The figure shows three views and two pictorial views of one solid part (mm, origin at its lowest corner). Answer the questions. Coordinates: 2 decimals unless noted, no trailing zeros. Write each loop counter-clockwise with the first axis right and the second up, starting at its lowest first coordinate (ties: lowest second). Pieces come first, ordered by that corner, then holes. Notation, with made-up numbers: (24, 57) - (41, 57) arc R11 cw to (41, 71) - close; hole circle Ø3 at (-32.5, -38). An arc over 180 degrees is marked (long way). Use a Markdown table: item, result. Add a question column.
(1) Given pin 1 Ø0.5 at (x, y) = (20.5, 0.5) entering from -Z; pin 2 Ø2.5 at (x, z) = (32.4, 18.17) entering from +Y; pin 3 Ø1.3 at (x, z) = (1.84, 1.84) entering from -Y; pin 4 Ø2 at (y, z) = (1.5, 2) entering from -X, each flat-ended and moving along its own axis, determine where each tip first touches the part or whether it passes through.
(2) The part is cut by section B-B, the plane x = 13. Give the vertices of the cut face in (y, z).
(3) The part is cut by section A-A, the plane y = 0.6. Give the vertices of the cut face in (x, z), then the cut area to 3 significant figures.
(4) Find the intervals of material crossed by line 1 (X direction, y = 0.4, z = 1) (1 decimal); line 2 (X direction, y = 0.6, z = 2.25) (1 decimal); line 3 (Y direction, x = 7, z = 12), in increasing order. Write a range as from..to.
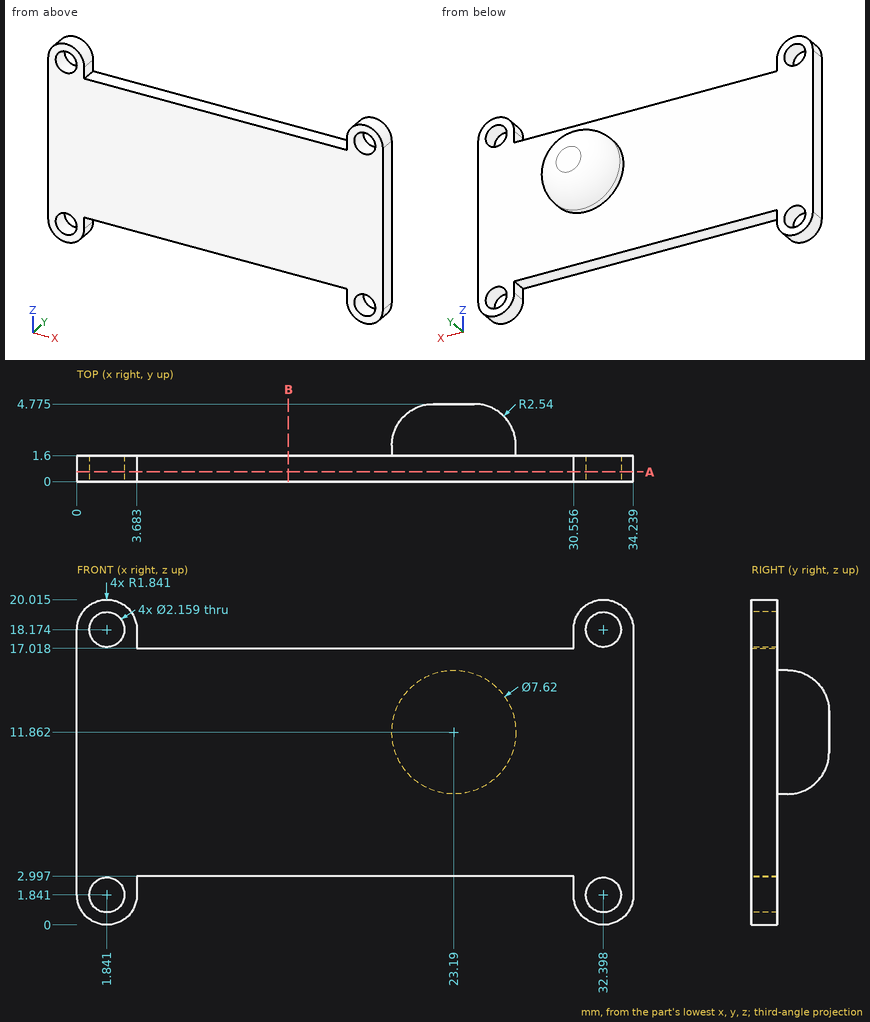
Model answer:
| question | item | result |
|---|---|---|
| 1 | pin 1 | z = 3 |
| 1 | pin 2 | y = 1.6 |
| 1 | pin 3 | through |
| 1 | pin 4 | x = 0 |
| 2 | outline | (0, 3) - (1.6, 3) - (1.6, 17.02) - (0, 17.02) - close |
| 3 | outline | (0, 1.84) arc R1.84 ccw to (3.68, 1.84) - (3.68, 3) - (30.56, 3) - (30.56, 1.84) arc R1.84 ccw to (34.24, 1.84) - (34.24, 18.17) arc R1.84 ccw to (30.56, 18.17) - (30.56, 17.02) - (3.68, 17.02) - (3.68, 18.17) arc R1.84 ccw to (0, 18.17) - close; hole circle Ø2.16 at (1.84, 1.84); hole circle Ø2.16 at (1.84, 18.17); hole circle Ø2.16 at (32.4, 1.84); hole circle Ø2.16 at (32.4, 18.17) |
| 3 | area | 504 mm^2 |
| 4 | line 1 | 0.2..1.2, 2.5..3.5, 30.8..31.7, 33.1..34 |
| 4 | line 2 | 0..0.8, 2.8..3.7, 30.6..31.4, 33.4..34.2 |
| 4 | line 3 | 0..1.6 |
